Can you work these out from the model? Positions are in its coordinate system, mm. A direction names the side the tool comes from. Round coordinates to 2 decimals unless told otherwise and drop trailing zeros. Order: outer loops, then holes, each group sorted by start corner. A loop starts at its lowest first (then second) coordinate and runs counter-clockwise, first axis right, second up. Notation, with made-up numbers: M 83,-36.5 L 115,-36.5 A24 cw 115,-14.5 Z; hole C 80.25,31 d3. An arc over 180 degrees is marked long. One line per question, with ' | ' between items.
```python
from build123d import *

# Parameters (mm, degrees)
F0_R     = 25.4
F1_DEPTH = 304.8
F1_TAPER = -3
F2_R     = 6.35
F3_T     = -2.54


with BuildPart() as f1:
    # F0 (on Top) → F1 (new body)
    with BuildSketch(Plane.XY):
        Circle(F0_R)
    extrude(amount=F1_DEPTH, taper=F1_TAPER)

    # F2
    f2_edges = [f1.edges().sort_by_distance(p)[0] for p in [
        (-25.4, 0, 0),
    ]]
    fillet(f2_edges, radius=F2_R)

    # F3
    f3_openings = [f1.faces().sort_by_distance(p)[0] for p in [
        (0, 0, 304.8),
    ]]
    offset(amount=F3_T, openings=f3_openings, kind=Kind.INTERSECTION)


solid = f1.part
```
(1) If we section it at A-A on x = 0: Please give me the cut outline in (y, z).
Final values:
outline: M -41.37,304.8 L -25.72,6.02 A6.35 ccw -19.37,0 L 19.37,0 A6.35 ccw 25.72,6.02 L 41.37,304.8 L 38.83,304.8 L 23.18,6.15 A3.81 cw 19.37,2.54 L -19.37,2.54 A3.81 cw -23.18,6.15 L -38.83,304.8 Z
(2) Please list where these lines run through material, in increasing order: probe 1 along Y at (x, z) = (-15, 236); probe 2 along Y at (x, z) = (6.5, 86); probe 3 along Z at (x, y) = (-1.5, -8). Write a range as [from, to].
Final values:
probe 1: [-34.66, -31.87], [31.87, 34.66] | probe 2: [-29.19, -26.58], [26.58, 29.19] | probe 3: [0, 2.54]
(3) Will these pins go through, and if not, where does the flat tip stop? pin 1 Ø1 at (x, y) = (15, -7) entering from +Z; pin 2 Ø6 at (y, z) = (-15, 35.5) entering from +X; pin 3 Ø1 at (x, z) = (8.5, 80.5) entering from +Y.
Final values:
pin 1: z = 2.54 | pin 2: x = 24.49 | pin 3: y = 28.52
(4) Thinking about a two-plate mould opening in Y: for faces 3 (the conical face through (14.357, -27.604, 157.566)), 4 (the flat face through (0, 0, 0)), 5 (the conical face through (32.1, 10.11, 157.5)), which applies, released by +Y, released by -Y, zero draft, split by the parting line, or undercut?
Final values:
face 3: undercut | face 4: zero draft | face 5: split by the parting line
(5) If we section it at B-B on z = 230: Please give me the cut outline in (x, y).
Final values:
outline: C 0,0 d74.91; hole C 0,0 d69.82
(6) On a 3-axis mill with a long thin cutter (end or side, diameter ignored), from which of +Z, -Z, +X, -X, +Y, -Y can I reach the whole of each face in a straight line? I mean faces 1 (the flat face through (0, 0, 2.54)), 2 (the flat face through (-12.5, 37, 304.8)). Say none if no direction works.
Final values:
face 1: +Z | face 2: +Z, +X, -X, +Y, -Y
(7) If we section it at C-C on z = 280.5: Please give me the cut outline in (x, y), plus the area to 3 significant figures.
Final values:
outline: C 0,0 d80.2; hole C 0,0 d75.11 | area: 621 mm^2
